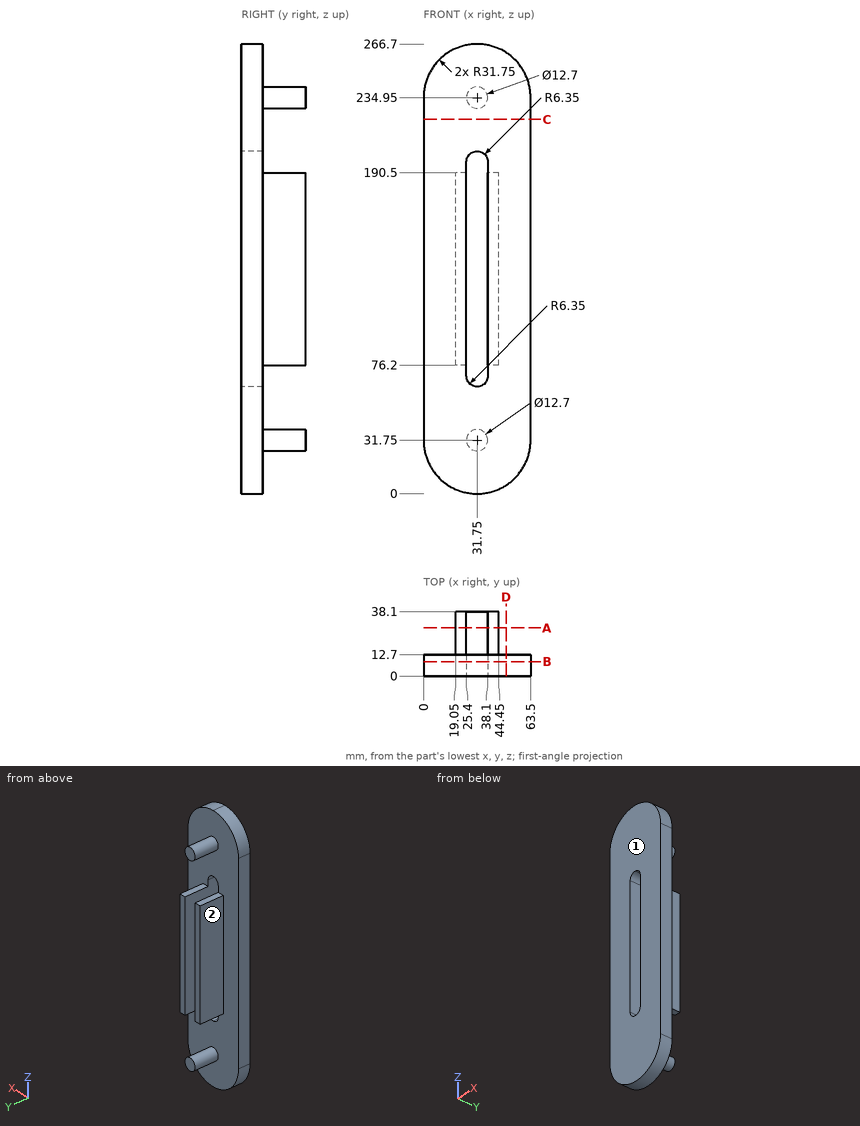
Could you check a few things on this drawing? It's one solid part, dimensions in mm from its lowest x, y, z. A direction names the side the tool comes from. Give positions to 0.01 mm unless a question says otherwise; leave off trailing zeros. Loops run counter-clockwise (first coordinate to the right, second up) from the corner with the lowest first, then second, coordinate; pieces in that order, holes last. Notation, with made-up numbers: M 85.5,58.25 L 123.5,58.25 A17 cw 123.5,65.25 Z; hole C -37.75,73.5 d2. An arc over 180 degrees is marked long. Answer as a JSON object with one key per item and string values.
Q1. For the marked faces 1 and 2, which set-ups out of +Z, -Z, +X, -X, +Y, -Y let a thin tool reach every point of the face, with its end or its side?
Values found:
{"face 1": "+Z, -Z, +X, -X, -Y", "face 2": "+Z, -Z, -X, +Y"}
Q2. Suppose I cut it at B-B, the plane y = 8.5. List the corners of the cut face in (x, z) for me.
Values found:
{"outline": "M 0,31.75 A31.75 ccw 63.5,31.75 L 63.5,234.95 A31.75 ccw 0,234.95 Z; hole M 25.4,69.85 A6.35 ccw 38.1,69.85 L 38.1,196.85 A6.35 ccw 25.4,196.85 Z"}
Q3. Suppose I cut it at C-C, the plane z = 222. List the corners of the cut face in (x, y) for me, plus the area to 3 significant figures.
Values found:
{"outline": "M 0,0 L 63.5,0 L 63.5,12.7 L 0,12.7 Z", "area": "806 mm²"}
Q4. If I drill on probe 1 along X at (y, z) = (5, 169.5); probe 2 along X at (y, z) = (13, 108); probe 3 along Y at (x, z) = (19.5, 65.5), over which ranges is the centre line in solid material (lowest first)? Write a range as [from, to].
Values found:
{"probe 1": "x = [0, 25.4], [38.1, 63.5]", "probe 2": "x = [19.05, 25.4], [38.1, 44.45]", "probe 3": "y = [0, 12.7]"}
Q5. For P1, Ø12, axis at x = 55.5, y = 21, coming from the +Z side; P2, Ø1.9, axis at x = 40.5, y = 31, coming from the +Z side; P3, Ø3, axis at x = 42, y = 31, coming from the -Z side; P4, Ø12, axis at y = 21.5, z = 86.5, coming from the -X side, each with a flat end and sliding along its axis, tell me the tip position at first contact or that it passes through.
Values found:
{"P1": "passes through", "P2": "stops at z = 190.5", "P3": "stops at z = 76.2", "P4": "stops at x = 19.05"}
Q6. Suppose I cut it at A-A, the plane y = 28.5. List the corners of the cut face in (x, z) for me.
Values found:
{"outline": "M 19.05,76.2 L 25.4,76.2 L 25.4,190.5 L 19.05,190.5 Z; C 31.75,31.75 d12.7; C 31.75,234.95 d12.7; M 38.1,76.2 L 44.45,76.2 L 44.45,190.5 L 38.1,190.5 Z"}
Q7. Suppose I cut it at D-D, the plane x = 49. List the corners of the cut face in (y, z) for me, plus the area to 3 significant figures.
Values found:
{"outline": "M 0,5.09 L 12.7,5.09 L 12.7,261.61 L 0,261.61 Z", "area": "3,260 mm²"}
